from build123d import *

# Parameters (mm, degrees)
SKETCH1_R           = 8.6995
SKETCH1_R_2         = 4.953
BOSS_EXTRUDE1_DEPTH = 2.794
CUT_EXTRUDE1_START  = -0.508
CUT_EXTRUDE1_DEPTH  = 0.508


with BuildPart() as part:
    # Sketch1 → Boss-Extrude1 (new body)
    with BuildSketch(Plane.XY):
        Circle(SKETCH1_R)
        Circle(SKETCH1_R_2, mode=Mode.SUBTRACT)
    extrude(amount=BOSS_EXTRUDE1_DEPTH)

    # Sketch2 → Cut-Extrude1 (cut)
    with BuildSketch(Plane.XY.offset(2.794).offset(CUT_EXTRUDE1_START)):
        with BuildLine():
            Line((7.385695624, 2.064428831), (8.303636404, 2.594402188))
            ThreePointArc((8.303636404, 2.594402188), (8.6995, 0), (8.303636405, -2.594402188))
            Line((8.303636405, -2.594402188), (7.385695624, -2.064428831))
            ThreePointArc((7.385695624, -2.064428831), (7.175606504, -1.831092109), (7.142804852, -1.518830175))
            ThreePointArc((7.142804852, -1.518830175), (7.3025, 0), (7.142804852, 1.518830175))
            ThreePointArc((7.142804852, 1.518830175), (7.175606504, 1.831092109), (7.385695624, 2.064428831))
        make_face()
        with BuildLine():
            Line((5.480695624, -5.363985619), (6.398636405, -5.893958976))
            ThreePointArc((6.398636405, -5.893958976), (4.34975, -7.533988), (1.905, -8.488361164))
            Line((1.905, -8.488361164), (1.905, -7.428414451))
            ThreePointArc((1.905, -7.428414451), (2.002030969, -7.129803575), (2.256056911, -6.945265543))
            ThreePointArc((2.256056911, -6.945265543), (3.65125, -6.324150511), (4.886747941, -5.426435369))
            ThreePointArc((4.886747941, -5.426435369), (5.173575535, -5.298711465), (5.480695624, -5.363985619))
        make_face()
        with BuildLine():
            Line((-1.905, -7.428414451), (-1.905, -8.488361164))
            ThreePointArc((-1.905, -8.488361164), (-4.34975, -7.533988), (-6.398636404, -5.893958976))
            Line((-6.398636404, -5.893958976), (-5.480695624, -5.36398562))
            ThreePointArc((-5.480695624, -5.36398562), (-5.173575535, -5.298711465), (-4.886747941, -5.426435369))
            ThreePointArc((-4.886747941, -5.426435369), (-3.65125, -6.324150511), (-2.256056911, -6.945265543))
            ThreePointArc((-2.256056911, -6.945265543), (-2.002030969, -7.129803575), (-1.905, -7.428414451))
        make_face()
        with BuildLine():
            Line((-7.385695624, -2.064428831), (-8.303636404, -2.594402188))
            ThreePointArc((-8.303636404, -2.594402188), (-8.6995, 0), (-8.303636405, 2.594402188))
            Line((-8.303636405, 2.594402188), (-7.385695624, 2.064428831))
            ThreePointArc((-7.385695624, 2.064428831), (-7.175606504, 1.831092109), (-7.142804852, 1.518830175))
            ThreePointArc((-7.142804852, 1.518830175), (-7.3025, 0), (-7.142804852, -1.518830175))
            ThreePointArc((-7.142804852, -1.518830175), (-7.175606504, -1.831092109), (-7.385695624, -2.064428831))
        make_face()
        with BuildLine():
            Line((-5.480695624, 5.363985619), (-6.398636405, 5.893958976))
            ThreePointArc((-6.398636405, 5.893958976), (-4.34975, 7.533988), (-1.905, 8.488361164))
            Line((-1.905, 8.488361164), (-1.905, 7.428414451))
            ThreePointArc((-1.905, 7.428414451), (-2.002030969, 7.129803575), (-2.256056911, 6.945265543))
            ThreePointArc((-2.256056911, 6.945265543), (-3.65125, 6.324150511), (-4.886747941, 5.426435369))
            ThreePointArc((-4.886747941, 5.426435369), (-5.173575535, 5.298711465), (-5.480695624, 5.363985619))
        make_face()
        with BuildLine():
            Line((6.398636404, 5.893958976), (5.480695624, 5.36398562))
            ThreePointArc((5.480695624, 5.36398562), (5.173575535, 5.298711465), (4.886747941, 5.426435369))
            ThreePointArc((4.886747941, 5.426435369), (3.65125, 6.324150511), (2.256056911, 6.945265543))
            ThreePointArc((2.256056911, 6.945265543), (2.002030969, 7.129803575), (1.905, 7.428414451))
            Line((1.905, 7.428414451), (1.905, 8.488361164))
            ThreePointArc((1.905, 8.488361164), (4.34975, 7.533988), (6.398636404, 5.893958976))
        make_face()
    extrude(amount=CUT_EXTRUDE1_DEPTH, mode=Mode.SUBTRACT)


solid = part.part
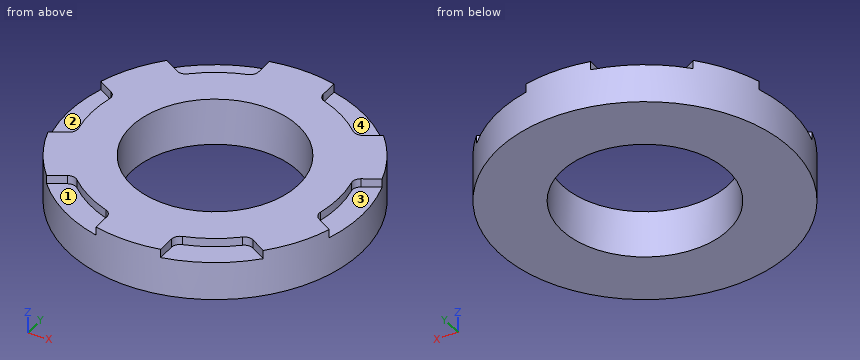
For this review, take the finished solid that the model builds, in its own axes (mm). Face numbers are marked on the shaded views. A direction names the side the tool comes from. Coordinates: 2 decimals unless noted, no trailing zeros. Write each loop counter-clockwise with the first axis right and the second up, starting at its lowest first coordinate (ties: lowest second). Pieces come first, ordered by that corner, then holes. Notation, with made-up numbers: (73, 65) -> (91, 65) arc R22 cw to (91, 75) -> close; hole circle Ø1 at (17.5, 13). An arc over 180 degrees is marked (long way). Write each question's results on one line, items separated by ' | '. Start each with the question number.
1) Wall thickness on L1, parallel to Y at x = 0, z = 2.1; L2, parallel to Z at x = -3.75, y = -7; L3, parallel to X at y = 3.25, z = 0.5: over which ranges is each line inside the solid? List them lowest first. Write a range as [from, to].
2) Consider section B-B (x = 0). Write out the cut boundary in (y, z).
3) Consider section D-D (x = 2.75). Write out the cut boundary in (y, z).
4) Consider section C-C (z = 1.1). Write out the cut boundary in (x, y), plus the area to 3 significant figures.
5) Insertion check: pin 1 (1.6 mm diameter, centred on x = 4, y = 7.5, fed in from +Z); pin 2 (1.5 mm diameter, centred on y = -3.5, z = 1.5, fed in from +X); pin 3 (6 mm diameter, centred on x = 1, y = -0.5, fed in from -Z). Each pin has a flat end and moves straight along its axis. Give the tip position at first contact, or say it passes through.
6) For the marked faces 1, 2, 3 and 4, list the 3-axis set-ups (+Z, -Z, +X, -X, +Y, -Y) from which the entire face can be reached by the end or side of a thin tool; tool diameter is ignored.
7) Consider section A-A (y = 0). Write out the cut boundary in (x, z), plus the area to 3 significant figures.
Geometry says:
1) L1: [-8.7, -4.95], [4.95, 8.7] | L2: [0, 2.29] | L3: [-8.07, -3.74], [3.74, 8.07]
2) outline: (-8.7, 0) -> (-4.95, 0) -> (-4.95, 2.79) -> (-8.7, 2.79) -> close; (4.95, 0) -> (8.7, 0) -> (8.7, 2.79) -> (4.95, 2.79) -> close
3) outline: (-8.25, 0) -> (-4.12, 0) -> (-4.12, 2.79) -> (-6.76, 2.79) -> (-6.76, 2.29) -> (-8.25, 2.29) -> close; (4.12, 0) -> (8.25, 0) -> (8.25, 2.29) -> (6.76, 2.29) -> (6.76, 2.79) -> (4.12, 2.79) -> close
4) outline: circle Ø17.4 at (0, 0); hole circle Ø9.91 at (0, 0) | area: 161 mm^2
5) pin 1: z = 2.29 | pin 2: x = 8.25 | pin 3: through
6) face 1: +Z, -Y | face 2: +Z, -X | face 3: +Z, +X | face 4: +Z, +Y
7) outline: (-8.7, 0) -> (-4.95, 0) -> (-4.95, 2.79) -> (-7.3, 2.79) -> (-7.3, 2.29) -> (-8.7, 2.29) -> close; (4.95, 0) -> (8.7, 0) -> (8.7, 2.29) -> (7.3, 2.29) -> (7.3, 2.79) -> (4.95, 2.79) -> close | area: 19.5 mm^2
